The model under review builds one solid part; all positions refer to its coordinate system, in mm. Face numbers are marked on the shaded views. A direction names the side the tool comes from. Coordinates: 2 decimals unless noted, no trailing zeros. Loops run counter-clockwise (first coordinate to the right, second up) from the corner with the lowest first, then second, coordinate; pieces in that order, holes last. Notation, with made-up numbers: M 6,-15 L 35,-15 A30 ccw 35,21 Z; hole C 69,2 d11. An arc over 180 degrees is marked long. One line per item, written item: value.
```python
from build123d import *

# Parameters (mm, degrees)
SZKIC1_R                    = 40
DODANIE_WYCI_GNI_CIE1_DEPTH = 22
SFAZOWANIE1_SIZE            = 2
SZKIC2_R                    = 55
DODANIE_WYCI_GNI_CIE2_DEPTH = 30


with BuildPart() as part:
    # Szkic1 → Dodanie-wyciągnięcie1 (new body)
    with BuildSketch(Plane(origin=(0, 0, 0), x_dir=(1, 0, 0), z_dir=(0, 1, 0))):
        with Locations(Location((0, 0, 0), (0, 0, 270))):
            Circle(SZKIC1_R)
        Polygon((-15.877132403, 27.5), (15.877132403, 27.5), (31.754264805, 0), (15.877132403, -27.5), (-15.877132403, -27.5), (-31.754264805, 0), align=None, mode=Mode.SUBTRACT)
    extrude(amount=DODANIE_WYCI_GNI_CIE1_DEPTH)

    # Sfazowanie1
    sfazowanie1_edges = [part.edges().sort_by_distance(p)[0] for p in [
        (-23.815698604, 22, -13.75),
        (-23.815698604, 22, 13.75),
        (0, 22, 27.5),
        (23.815698604, 22, 13.75),
        (23.815698604, 22, -13.75),
        (0, 22, -27.5),
    ]]
    chamfer(sfazowanie1_edges, length=SFAZOWANIE1_SIZE)

    # Szkic2 → Dodanie-wyciągnięcie2 (add)
    with BuildSketch(Plane.XZ):
        with Locations(Location((0, 0, 0), (0, 0, 270))):
            Circle(SZKIC2_R)
    extrude(amount=DODANIE_WYCI_GNI_CIE2_DEPTH)


solid = part.part
```
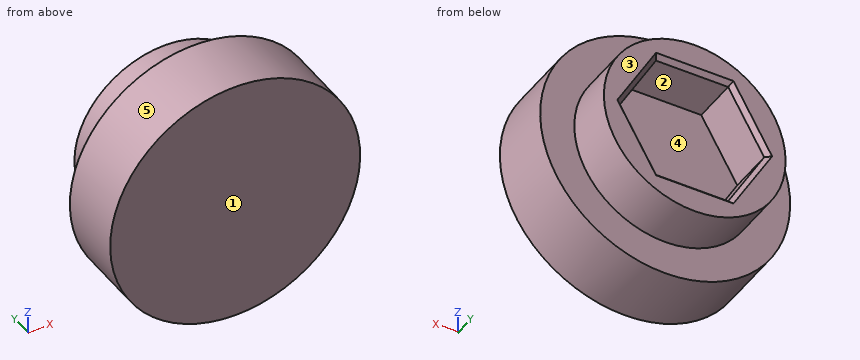
(1) Add section A-A on x = 0. State the section outline as (y, z) points.
Checks:
outline: M -30,-55 L 0,-55 L 0,-40 L 22,-40 L 22,-29.5 L 20,-27.5 L 0,-27.5 L 0,27.5 L 20,27.5 L 22,29.5 L 22,40 L 0,40 L 0,55 L -30,55 Z
(2) Add section C-C on y = -11.5. State the section outline as (x, z) points, then the cut area to 3 significant figures.
Checks:
outline: C 0,0 d110
area: 9,500 mm^2
(3) Add section D-D on x = 37. State the section outline as (y, z) points.
Checks:
outline: M -30,-40.69 L 0,-40.69 L 0,-15.2 L 22,-15.2 L 22,15.2 L 0,15.2 L 0,40.69 L -30,40.69 Z
(4) Tool access review of the marked faces 1 and 2: name each direction out of +Z, -Z, +X, -X, +Y, -Y from which nothing blocks a thin tool from reaching the whole face with its end or side.
Checks:
face 1: +Z, -Z, +X, -X, -Y
face 2: +Y
(5) Draft analysis for pull direction X (two halves, no side actions). For the marked faces 3, 4 and 5, state which applies: pulls with the +X half, pulls with the -X half, needs draft (parallel to the pull), parting line crosses it, or undercut.
Checks:
face 3: needs draft
face 4: undercut
face 5: parting line crosses it
(6) Add section B-B on z = -13.5. State the section outline as (x, y) points.
Checks:
outline: M -53.32,-30 L 53.32,-30 L 53.32,0 L 37.65,0 L 37.65,22 L 26.27,22 L 23.96,20 L 23.96,0 L -23.96,0 L -23.96,20 L -26.27,22 L -37.65,22 L -37.65,0 L -53.32,0 Z
(7) To check wall thickness, follow L1, parallel to Z at x = 1, y = 5; L2, parallel to Y at x = 17, z = 23; L3, parallel to X at y = 8.5, z = 15. State the ranges of each line that lie inside material, in increasing order. Write a range as [from, to].
Checks:
L1: [-39.99, -27.5], [27.5, 39.99]
L2: [-30, 0]
L3: [-37.08, -23.09], [23.09, 37.08]
(8) Insertion check: pin 1 Ø6 at (x, y) = (-15, 0.5) entering from +Z; pin 2 Ø5 at (y, z) = (7.5, 24) entering from -X; pin 3 Ø10 at (y, z) = (2, -10) entering from -X. Each pin has a flat end and moves straight along its axis. Give the tip position at first contact, or say it passes through.
Checks:
pin 1: z = 53.67
pin 2: x = -33.73
pin 3: x = -54.73
